```python
from build123d import *

# Parameters (mm, degrees)
F1_ANGLE = 60


# Not quite as in the source:
# - a feature of the source that left no trace in its solid (it failed there, or was rolled back) is left out


with BuildPart() as f1:
    # F0 (on Front) → F1 (revolve)
    with BuildSketch(Plane.XZ):
        with BuildLine():
            Line((-15.24, 0), (0, 0))
            Line((0, 0), (0, 50.8))
            Line((0, 50.8), (-6.35, 50.8))
            Line((-6.35, 50.8), (-4.7617064118, 41.792339449))
            ThreePointArc((-4.7617064118, 41.792339449), (-4.8311637627, 41.5331210865), (-5.0743828734, 41.4197061526))
            Line((-5.0743828734, 41.4197061526), (-6.2835011077, 41.4197061526))
            ThreePointArc((-6.2835011077, 41.4197061526), (-6.5080075107, 41.3267125556), (-6.6010011077, 41.1022061526))
            Line((-6.6010011077, 41.1022061526), (-6.6010011077, 40.4672061526))
            ThreePointArc((-6.6010011077, 40.4672061526), (-6.5080075107, 40.2426997495), (-6.2835011077, 40.1497061526))
            Line((-6.2835011077, 40.1497061526), (-5.0743828734, 40.1497061526))
            ThreePointArc((-5.0743828734, 40.1497061526), (-4.8311637627, 40.0362912186), (-4.7617064118, 39.7770728561))
            Line((-4.7617064118, 39.7770728561), (-5.2010717431, 37.2853082403))
            ThreePointArc((-5.2010717431, 37.2853082403), (-5.3096631386, 37.0972224261), (-5.5137482047, 37.0229415367))
            Line((-5.5137482047, 37.0229415367), (-6.8348340718, 37.0229415367))
            ThreePointArc((-6.8348340718, 37.0229415367), (-7.0593404748, 36.9299479398), (-7.1523340718, 36.7054415367))
            Line((-7.1523340718, 36.7054415367), (-7.1523340718, 36.0704415367))
            ThreePointArc((-7.1523340718, 36.0704415367), (-7.2453276688, 35.8459351337), (-7.4698340718, 35.7529415367))
            Line((-7.4698340718, 35.7529415367), (-8.7398340718, 35.7529415367))
            ThreePointArc((-8.7398340718, 35.7529415367), (-8.9643404748, 35.6599479398), (-9.0573340718, 35.4354415367))
            Line((-9.0573340718, 35.4354415367), (-9.0573340718, 34.8004415367))
            ThreePointArc((-9.0573340718, 34.8004415367), (-8.9643404748, 34.5759351337), (-8.7398340718, 34.4829415367))
            Line((-8.7398340718, 34.4829415367), (-3.5686493249, 34.4829415367))
            ThreePointArc((-3.5686493249, 34.4829415367), (-3.3254302142, 34.3695266028), (-3.2559728633, 34.1103082403))
            Line((-3.2559728633, 34.1103082403), (-7.113602572, 12.2326030065))
            ThreePointArc((-7.113602572, 12.2326030065), (-7.2221939675, 12.0445171922), (-7.4262790336, 11.9702363029))
            Line((-7.4262790336, 11.9702363029), (-8.1123649007, 11.9702363029))
            ThreePointArc((-8.1123649007, 11.9702363029), (-8.3368713037, 11.8772427059), (-8.4298649007, 11.6527363029))
            Line((-8.4298649007, 11.6527363029), (-8.4298649007, 8.9432889844))
            ThreePointArc((-8.4298649007, 8.9432889844), (-8.4596121783, 8.8091076862), (-8.5432798346, 8.7000698737))
            Line((-8.5432798346, 8.7000698737), (-15.1265850661, 3.176020882))
            ThreePointArc((-15.1265850661, 3.176020882), (-15.2102527224, 3.0669830694), (-15.24, 2.9328017713))
            Line((-15.24, 2.9328017713), (-15.24, 0))
        make_face()
    revolve(axis=Axis((0, 0, 25.4), (0, 0, 1)), revolution_arc=F1_ANGLE)


solid = f1.part
```
Verification items for the finished model (mm, model axes). A direction names the side the tool comes from. Coordinates: 2 decimals unless noted, no trailing zeros. Write each loop counter-clockwise with the first axis right and the second up, starting at its lowest first coordinate (ties: lowest second). Pieces come first, ordered by that corner, then holes. Notation, with made-up numbers: M 19.5,-19 L 24.5,-19 A6 ccw 24.5,-14 Z; hole C 31.25,81.25 d8. An arc over 180 degrees is marked long. Answer as a JSON object with one key per item and string values. Group by question number.
(1) Release check for a two-part mould opening along Z. For faces 4 (the face through (-9, -5, 0)), 5 (the face through (-6.22, -3.53, 36.38)), 6 (the face through (-3, -2, 50.8)), 7 (the face through (-7.33, -4.16, 10.28)) record: +Z half, -Z half, draft (parallel to the pull), parting line (faces both ways), or undercut.
(2) Cross-section at A-A, the plane z = 10. Record the cut outline in (x, y), and give its area (3 significant figures).
(3) Gauge pin test, flat ends, axial feed: pin 1 (1.3 mm diameter, centred on x = -5.5, y = -5, fed in from +Z); pin 2 (6 mm diameter, centred on x = -6.5, z = 13, fed in from -Y); pin 3 (3 mm diameter, centred on x = -6.5, z = 10, fed in from -Y); pin 4 (1.5 mm diameter, centred on y = -8, z = 32.5, fed in from -X). Record the tip position at first contact, or that the pin passes through.
(4) Cross-section at B-B, the plane z = 29.5. Record the cut outline in (x, y).
(5) Tool access check on faces 1 (the face through (-7, -4, 35.753)), 2 (the face through (-5, -3, 41.42)), 3 (the face through (-4, 0, 20)). Record the directions out of +Z, -Z, +X, -X, +Y, -Y that give a thin tool (end or side, any length) a straight path to the whole face; none if there is none.
(6) Material ranges on line 1 (Y direction, x = -2.75, z = 8.5); line 2 (Z direction, x = -12.75, y = -7.5); line 3 (Z direction, x = -12, y = -2), recorded low to high.
Reply:
{
 "1": {"face 4": "-Z half", "face 5": "draft", "face 6": "+Z half", "face 7": "undercut"},
 "2": {"outline": "M -8.43,0 A8.43 ccw -4.21,-7.3 L 0,0 Z", "area": "37.2 mm²"},
 "3": {"pin 1": "z = 37.02", "pin 2": "y = -7.3", "pin 3": "y = -6.79", "pin 4": "through"},
 "4": {"outline": "M -4.07,0 A4.07 ccw -2.03,-3.52 L 0,0 Z"},
 "5": {"face 1": "+Z, -X, -Y", "face 2": "-X, -Y", "face 3": "+Z, -Z, +X, -X, +Y"},
 "6": {"line 1": "-4.76 to 0", "line 2": "0 to 3.46", "line 3": "0 to 5.66"}
}
